Input: part model. Units: mm. Frame: model coordinates. Round coordinates to 2 decimals unless told otherwise and drop trailing zeros. Loops run counter-clockwise (first coordinate to the right, second up) from the corner with the lowest first, then second, coordinate; pieces in that order, holes last.
1) Draft query along Z for faces 1 (the face through (9.1, 1, -8.7)), 2 (the face through (0.285, 1.014, -0.301)), 3 (the face through (0.285, 1.014, -14.699)). Return one class per face: pulls with the +Z half, pulls with the -Z half, needs draft (parallel to the pull), parting line crosses it, or undercut.
2) Section A-A, the plane x = 50. Return loops of the section in (y, z), and give its area (3 significant figures).
3) Section B-B, the plane z = -7.5. Return loops of the section in (x, y).
4) Section C-C, the plane y = 1. Return loops of the section in (x, z).
5) Ray query, line 1 along X through (y, z) = (1.1, -7.5); line 2 along Z through (x, y) = (51, 0.75); line 3 along X through (y, z) = (1.4, -0.25). Return the intervals inside material, ascending.
from build123d import *

# Parameters (mm, degrees)
SKETCH1_W           = 60
SKETCH1_H           = 15
SKETCH1_R           = 1.5
BOSS_EXTRUDE1_DEPTH = 2
FILLET1_R           = 1


with BuildPart() as part:
    # Sketch1 → Boss-Extrude1 (new body)
    with BuildSketch(Plane(origin=(0, 0, 0), x_dir=(1, 0, 0), z_dir=(0, 1, 0))):
        with Locations((30, 7.5)):
            Rectangle(SKETCH1_W, SKETCH1_H)
        with Locations(Location((50, 7.5, 0), (0, 0, 270))):
            Circle(SKETCH1_R, mode=Mode.SUBTRACT)
        with Locations(Location((10, 7.5, 0), (0, 0, 270))):
            Circle(SKETCH1_R, mode=Mode.SUBTRACT)
    extrude(amount=BOSS_EXTRUDE1_DEPTH)

    # Fillet1
    fillet1_edges = [part.edges().sort_by_distance(p)[0] for p in [
        (0, 1, 0),
        (0, 1, -15),
        (60, 1, -15),
        (60, 1, 0),
    ]]
    fillet(fillet1_edges, radius=FILLET1_R)


solid = part.part
Final values:
1. face 1: undercut
1. face 2: pulls with the +Z half
1. face 3: pulls with the -Z half
2. outline: (0, -15) - (2, -15) - (2, -9) - (0, -9) - close; (0, -6) - (2, -6) - (2, 0) - (0, 0) - close
2. area: 24.0 mm2
3. outline: (0, 0) - (8.5, 0) - (8.5, 2) - (0, 2) - close; (11.5, 0) - (48.5, 0) - (48.5, 2) - (11.5, 2) - close; (51.5, 0) - (60, 0) - (60, 2) - (51.5, 2) - close
4. outline: (0, -14) arc R1 ccw to (1, -15) - (59, -15) arc R1 ccw to (60, -14) - (60, -1) arc R1 ccw to (59, 0) - (1, 0) arc R1 ccw to (0, -1) - close; hole circle Ø3 at (10, -7.5); hole circle Ø3 at (50, -7.5)
5. line 1: x = 0 to 8.5, 11.5 to 48.5, 51.5 to 60
5. line 2: z = -15 to -8.62, -6.38 to 0
5. line 3: x = 0.34 to 59.66
